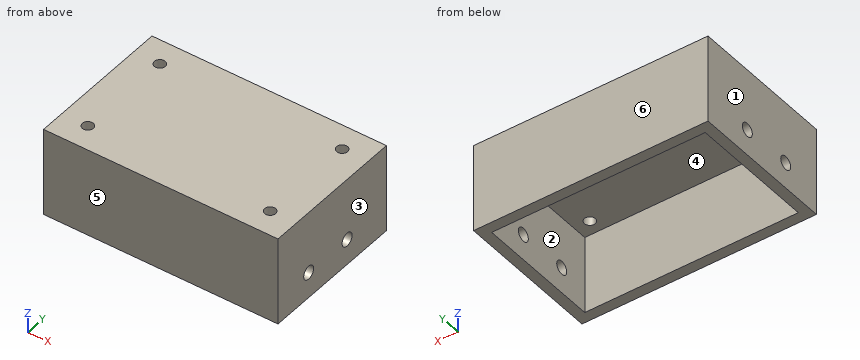
```python
from build123d import *

# Parameters (mm, degrees)
SKETCH1_W           = 5.08
SKETCH1_H           = 61.595
SKETCH1_W_2         = 104.14
SKETCH1_R           = 2.667
BOSS_EXTRUDE1_DEPTH = 5.08
SKETCH1_3_W         = 5.08
SKETCH1_3_H         = 61.595
BOSS_EXTRUDE2_DEPTH = 38.1
SKETCH2_R           = 3.302
CUT_EXTRUDE1_DEPTH  = 125.356688627
SKETCH3_W           = 114.3
SKETCH3_H           = 43.18
BOSS_EXTRUDE3_DEPTH = 5.08
BOSS_EXTRUDE4_START = -61.595
SKETCH3_3_W         = 114.3
SKETCH3_3_H         = 43.18
BOSS_EXTRUDE4_DEPTH = 5.08


with BuildPart() as part:
    # Sketch1 → Boss-Extrude1 (new body)
    # profile 1 of 3: a face of its own
    with BuildSketch(Plane.XY):
        with Locations((-54.61, 0)):
            Rectangle(SKETCH1_W, SKETCH1_H)
    # profile 2 of 3: a face of its own
    with BuildSketch(Plane.XY):
        Rectangle(SKETCH1_W_2, SKETCH1_H)
        with Locations((-44.45, -23.8125)):
            Circle(SKETCH1_R, mode=Mode.SUBTRACT)
        with Locations((44.45, -23.8125)):
            Circle(SKETCH1_R, mode=Mode.SUBTRACT)
        with Locations((-44.45, 23.8125)):
            Circle(SKETCH1_R, mode=Mode.SUBTRACT)
        with Locations((44.45, 23.8125)):
            Circle(SKETCH1_R, mode=Mode.SUBTRACT)
    # profile 3 of 3: a face of its own
    with BuildSketch(Plane.XY):
        with Locations((54.61, 0)):
            Rectangle(SKETCH1_W, SKETCH1_H)
    extrude(amount=BOSS_EXTRUDE1_DEPTH)

    # Sketch1<3> → Boss-Extrude2 (add)
    with BuildSketch(Plane.XY):
        with Locations((-54.61, 0)):
            Rectangle(SKETCH1_3_W, SKETCH1_3_H)
        with Locations((54.61, 0)):
            Rectangle(SKETCH1_3_W, SKETCH1_3_H)
    extrude(amount=-BOSS_EXTRUDE2_DEPTH)

    # Sketch2 → Cut-Extrude1 (cut, through all)
    with BuildSketch(Plane(origin=(57.15, 0, 0), x_dir=(0, 0, -1), z_dir=(1, 0, 0))):
        with Locations((25.4, -15.5575)):
            Circle(SKETCH2_R)
        with Locations((25.4, 9.8425)):
            Circle(SKETCH2_R)
    extrude(amount=-CUT_EXTRUDE1_DEPTH, mode=Mode.SUBTRACT)

    # Sketch3 → Boss-Extrude3 (add)
    with BuildSketch(Plane(origin=(0, 30.7975, 0), x_dir=(1, 0, 0), z_dir=(0, 1, 0))):
        with Locations((0, 16.51)):
            Rectangle(SKETCH3_W, SKETCH3_H)
    extrude(amount=BOSS_EXTRUDE3_DEPTH)

    # Sketch3<3> → Boss-Extrude4 (add)
    with BuildSketch(Plane(origin=(0, 30.7975, 0), x_dir=(1, 0, 0), z_dir=(0, 1, 0)).offset(BOSS_EXTRUDE4_START)):
        with Locations((0, 16.51)):
            Rectangle(SKETCH3_3_W, SKETCH3_3_H)
    extrude(amount=-BOSS_EXTRUDE4_DEPTH)


solid = part.part
```
Check sheet for the modelled part. Datum: model origin and axes. Units: mm. Face numbers are marked on the shaded views. A direction names the side the tool comes from. Round coordinates to 2 decimals unless told otherwise and drop trailing zeros. Order: outer loops, then holes, each group sorted by start corner. A loop starts at its lowest first (then second) coordinate and runs counter-clockwise, first axis right, second up. Notation, with made-up numbers: (28, 34.5) -> (84, 34.5) arc R27 cw to (84, 65.5) -> close; hole circle Ø8 at (66, 76.5). An arc over 180 degrees is marked (long way). Use CSV: the item, a comma, the result in double quotes.
(1) Material ranges on line 1 along Y through (x, z) = (55, -25); line 2 along Y through (x, z) = (22.5, -13.5); line 3 along X through (y, z) = (-30, -20.5), recorded low to high. Write a range as from..to.
Worked out:
line 1,"-35.88..-18.84, -12.28..6.56, 13.12..35.88"
line 2,"-35.88..-30.8, 30.8..35.88"
line 3,"-57.15..-52.07, 52.07..57.15"
(2) Tool access check on the marked faces 1 and 2. Record the directions out of +Z, -Z, +X, -X, +Y, -Y that give a thin tool (end or side, any length) a straight path to the whole face; none if there is none.
Worked out:
face 1,"+Z, -Z, -X, +Y, -Y"
face 2,"-Z"
(3) Cross-section at B-B (x = -44.45). Record the boundary of the cut face in (y, z).
Worked out:
outline,"(-35.88, -38.1) -> (-30.8, -38.1) -> (-30.8, 0) -> (-26.48, 0) -> (-26.48, 5.08) -> (-35.88, 5.08) -> close; (-21.15, 0) -> (21.15, 0) -> (21.15, 5.08) -> (-21.15, 5.08) -> close; (26.48, 0) -> (30.8, 0) -> (30.8, -38.1) -> (35.88, -38.1) -> (35.88, 5.08) -> (26.48, 5.08) -> close"
(4) Cross-section at D-D (z = -12). Record the boundary of the cut face in (x, y), and give its area (3 significant figures).
Worked out:
outline,"(-57.15, -35.88) -> (57.15, -35.88) -> (57.15, 35.88) -> (-57.15, 35.88) -> close; hole (-52.07, -30.8) -> (52.07, -30.8) -> (52.07, 30.8) -> (-52.07, 30.8) -> close"
area,"1,790 mm²"
(5) Cross-section at A-A (z = -25.4). Record the boundary of the cut face in (x, y), and give its area (3 significant figures).
Worked out:
outline,"(-57.15, -35.88) -> (57.15, -35.88) -> (57.15, -18.86) -> (52.07, -18.86) -> (52.07, -30.8) -> (-52.07, -30.8) -> (-52.07, -18.86) -> (-57.15, -18.86) -> close; (-57.15, -12.26) -> (-52.07, -12.26) -> (-52.07, 6.54) -> (-57.15, 6.54) -> close; (-57.15, 13.14) -> (-52.07, 13.14) -> (-52.07, 30.8) -> (52.07, 30.8) -> (52.07, 13.14) -> (57.15, 13.14) -> (57.15, 35.88) -> (-57.15, 35.88) -> close; (52.07, -12.26) -> (57.15, -12.26) -> (57.15, 6.54) -> (52.07, 6.54) -> close"
area,"1,650 mm²"
(6) Depth check by flat-ended pin: pin 1 (4 mm diameter, centred on y = 9.84, z = -25.4, fed in from +X); pin 2 (6 mm diameter, centred on x = 44.45, y = -23.81, fed in from -Z). Enter the tip coordinate at first touch or a pass-through.
Worked out:
pin 1,"through"
pin 2,"z = 0"
(7) Draft check along Y on the marked faces 3, 4, 5 and 6. Enter one of: pulls with the +Y half, pulls with the -Y half, needs draft (parallel to the pull), parting line crosses it, or undercut.
Worked out:
face 3,"needs draft"
face 4,"undercut"
face 5,"pulls with the -Y half"
face 6,"pulls with the +Y half"
(8) Cross-section at C-C (y = 29.5). Record the boundary of the cut face in (x, z), and give its area (3 significant figures).
Worked out:
outline,"(-57.15, -38.1) -> (-52.07, -38.1) -> (-52.07, 0) -> (52.07, 0) -> (52.07, -38.1) -> (57.15, -38.1) -> (57.15, 5.08) -> (-57.15, 5.08) -> close"
area,"968 mm²"
